Design review of the part built by this model. Coordinates are the model's own, in mm. A direction names the side the tool comes from. Round coordinates to 2 decimals unless told otherwise and drop trailing zeros. Order: outer loops, then holes, each group sorted by start corner. A loop starts at its lowest first (then second) coordinate and runs counter-clockwise, first axis right, second up. Notation, with made-up numbers: (-14.5, 89) - (-5.5, 89) arc R13 ccw to (-5.5, 106) - close; hole circle Ø3 at (34, -31). An arc over 180 degrees is marked (long way). Write item = value, one per line.
from build123d import *

# Parameters (mm, degrees)
F0_R     = 13
F0_R_2   = 11
F1_DEPTH = 7


with BuildPart() as f1:
    # F0 (on Top) → F1 (new body)
    with BuildSketch(Plane.XY):
        with BuildLine():
            Line((25, 15), (-25, 15))
            ThreePointArc((-25, 15), (-50, 0), (-25, -15))
            Line((-25, -15), (0, -15))
            Line((0, -15), (25, -15))
            ThreePointArc((25, -15), (50, 0), (25, 15))
        make_face()
        with Locations((-33, 0)):
            Circle(F0_R, mode=Mode.SUBTRACT)
        Circle(F0_R_2, mode=Mode.SUBTRACT)
        with Locations((33, 0)):
            Circle(F0_R, mode=Mode.SUBTRACT)
    extrude(amount=F1_DEPTH)


solid = f1.part
1) The part is to be moulded in two halves that separate along Y. For faces 1 (the cylindrical face through (-2.38, -10.74, 3.45)), 2 (the flat face through (0, -15, 3)), 3 (the cylindrical face through (-50, 0, 3)), say which applies: released by +Y, released by -Y, zero draft, split by the parting line, or undercut.
Findings:
face_1 = undercut
face_2 = released by -Y
face_3 = split by the parting line
2) We need section A-A on y = 0. Write out the cut boundary in (x, z).
Findings:
outline = (-50, 0) - (-46, 0) - (-46, 7) - (-50, 7) - close; (-20, 0) - (-11, 0) - (-11, 7) - (-20, 7) - close; (11, 0) - (20, 0) - (20, 7) - (11, 7) - close; (46, 0) - (50, 0) - (50, 7) - (46, 7) - close
3) To check wall thickness, follow L1, parallel to X at y = 0.5, z = 1.5; L2, parallel to Y at x = 33, z = 2.25; L3, parallel to X at y = -4.5, z = 2.5. State the ranges of each line that lie inside material, in increasing order. Write a range as from..to.
Findings:
L1 = -49.99..-45.99, -20.01..-10.99, 10.99..20.01, 45.99..49.99
L2 = -17..-13, 13..17
L3 = -49.39..-45.2, -20.8..-10.04, 10.04..20.8, 45.2..49.39
4) We need section C-C on z = 1.25. Write out the cut boundary in (x, y), and give its area (3 significant figures).
Findings:
outline = (-25, -15) - (25, -15) arc R17 ccw (long way) to (25, 15) - (-25, 15) arc R17 ccw (long way) to start; hole circle Ø26 at (-33, 0); hole circle Ø22 at (0, 0); hole circle Ø26 at (33, 0)
area = 1,490 mm^2
5) For faces 4 (the flat face through (-12, 0, 0)), 5 (the flat face through (0, 15, 3)), list the 3-axis set-ups (+Z, -Z, +X, -X, +Y, -Y) from which the entire face can be reached by the end or side of a thin tool; tool diameter is ignored.
Findings:
face_4 = -Z, +X, -X, +Y, -Y
face_5 = +Z, -Z, +Y
6) We need section D-D on x = -1. Write out the cut boundary in (y, z), and give its area (3 significant figures).
Findings:
outline = (-15, 0) - (-10.95, 0) - (-10.95, 7) - (-15, 7) - close; (10.95, 0) - (15, 0) - (15, 7) - (10.95, 7) - close
area = 56.6 mm^2
7) Clearance check with flat-ended pins moving along their axes: pin 1 Ø1.5 at (y, z) = (6, 3) entering from -X; pin 2 Ø1 at (y, z) = (-2, 2.5) entering from +X; pin 3 Ø2 at (x, z) = (-24.5, 2.5) entering from -Y. State where each tip first meets the part, or that it passes through.
Findings:
pin_1 = -49.17
pin_2 = 49.93
pin_3 = -15.26
8) We need section B-B on x = 33. Write out the cut boundary in (y, z).
Findings:
outline = (-17, 0) - (-13, 0) - (-13, 7) - (-17, 7) - close; (13, 0) - (17, 0) - (17, 7) - (13, 7) - close
